from build123d import *

# Parameters (mm, degrees)
F0_W     = 101.6
F0_H     = 38.1
F1_DEPTH = 101.6
F2_T     = -3.175
F4_D     = 7.9375
F4_DEPTH = 12.7
F4_TIP   = 2.3846655818
F3_W     = 13.1781175733
F3_H     = 4.8110592179
F5_DEPTH = 3.175


# Not quite as in the source:
# - a length typed as a fraction of an inch, garbled in the dataset ("3 / 203.2 mm" for 3/8 in), is restored


with BuildPart() as f1:
    # F0 (on Front) → F1 (new body)
    with BuildSketch(Plane.XZ):
        with Locations((10.0446864963, 7.5280469467)):
            Rectangle(F0_W, F0_H)
    extrude(amount=F1_DEPTH)

    # F2
    f2_openings = [f1.faces().sort_by_distance(p)[0] for p in [
        (10.044686, -50.8, 26.578047),
    ]]
    offset(amount=F2_T, openings=f2_openings)

    # F4
    with Locations(Plane.YZ.offset(60.8446864963)):
        with Locations((-17.720233649, 5.8569414541)):
            Hole(F4_D / 2, depth=F4_DEPTH)
            with Locations((0, 0, -(F4_DEPTH + F4_TIP / 2))):  # 118° drill point
                Cone(0, F4_D / 2, F4_TIP, mode=Mode.SUBTRACT)

    # F3 (on face) → F5 (cut, through all)
    with BuildSketch(Plane.YZ.offset(60.8446864963)):
        with Locations((-76.6034089029, 9.3083532993)):
            Rectangle(F3_W, F3_H)
    extrude(amount=-F5_DEPTH, mode=Mode.SUBTRACT)


solid = f1.part
Can you work these out from the model? Positions are in its coordinate system, mm. A direction names the side the tool comes from. Coordinates: 2 decimals unless noted, no trailing zeros. Write each loop counter-clockwise with the first axis right and the second up, starting at its lowest first coordinate (ties: lowest second). Pieces come first, ordered by that corner, then holes. Notation, with made-up numbers: M 47,43.25 L 78,43.25 A23 ccw 78,53.25 Z; hole C -8,-22.75 d9. An arc over 180 degrees is marked long. Use one line per item in the form item = value.
Q1. I need wall thicknesses on line 1 along Y through (x, z) = (-20.5, -7) (3 decimals); line 2 along X through (y, z) = (-20, 14.5); line 3 along Z through (x, y) = (-3, -39). Which ranges of each line are inside material? Lowest first, please. Write a range as from..to.
Model answer:
line_1 = -101.6..-98.425, -3.175..0
line_2 = -40.76..-37.58, 57.67..60.84
line_3 = -11.52..-8.35
Q2. If we section it at D-D (y = -26.5): Write out the boundary of the cut face in (x, z).
Model answer:
outline = M -40.76,-11.52 L 60.84,-11.52 L 60.84,26.58 L 57.67,26.58 L 57.67,-8.35 L -37.58,-8.35 L -37.58,26.58 L -40.76,26.58 Z
Q3. We'd pull the mould along Y, two halves only. Please class faces 4 (the cylindrical face through (59.235, -14.795, 8.539)), 5 (the flat face through (-40.755, -50, 7)), 6 (the flat face through (9, -101.6, 8)): +Y half, -Y half, draft (parallel to the pull), parting line (faces both ways), or undercut.
Model answer:
face_4 = undercut
face_5 = draft
face_6 = -Y half
Q4. For P1, Ø6, axis at x = 38, z = 13.5, coming from the +Y side; P2, Ø12, axis at x = -27, y = -49, coming from the +Z side, each with a flat end and sliding along its axis, tell me the tip position at first contact or that it passes through.
Model answer:
P1 = 0
P2 = -8.35
Q5. For faces 1 (the flat face through (6, -99, 26.578)), 2 (the flat face through (59, -77, 6.903)), 3 (the flat face through (9, -3.175, 9)), which set-ups out of +Z, -Z, +X, -X, +Y, -Y let a thin tool reach every point of the face, with its end or its side?
Model answer:
face_1 = +Z, +X, -X, +Y, -Y
face_2 = +X
face_3 = +Z
Q6. If we section it at A-A (y = -79): Write out the boundary of the cut face in (x, z).
Model answer:
outline = M -40.76,-11.52 L 60.84,-11.52 L 60.84,6.9 L 57.67,6.9 L 57.67,-8.35 L -37.58,-8.35 L -37.58,26.58 L -40.76,26.58 Z; M 57.67,11.71 L 60.84,11.71 L 60.84,26.58 L 57.67,26.58 Z
Q7. If we section it at B-B (z = 17.5): Write out the boundary of the cut face in (x, y) (3 decimals).
Model answer:
outline = M -40.755,-101.6 L 60.845,-101.6 L 60.845,0 L -40.755,0 Z; hole M -37.58,-98.425 L 57.67,-98.425 L 57.67,-3.175 L -37.58,-3.175 Z
Q8. If we section it at C-C (x = -32): Write out the boundary of the cut face in (y, z) (3 decimals).
Model answer:
outline = M -101.6,-11.522 L 0,-11.522 L 0,26.578 L -3.175,26.578 L -3.175,-8.347 L -98.425,-8.347 L -98.425,26.578 L -101.6,26.578 Z
